Geometry: final body of the model. Coordinates: model frame, mm. A direction names the side the tool comes from. Coordinates: 2 decimals unless noted, no trailing zeros. Order: outer loops, then holes, each group sorted by start corner. A loop starts at its lowest first (then second) coordinate and runs counter-clockwise, first axis right, second up. Notation, with made-up numbers: (43, 74.25) - (68, 74.25) arc R25 ccw to (68, 113.25) - close; hole circle Ø4 at (64.5, -22.75). An arc over 180 degrees is marked (long way). Use a Markdown table: item, result. Add a question column.
```python
from build123d import *

# Parameters (mm, degrees)
ESBO_O1_W                = 77
ESBO_O1_H                = 57.5
RESSALTO_EXTRUS_O1_DEPTH = 2
ESBO_O2_W                = 7.7755798
ESBO_O2_H                = 8.143597904
ESBO_O2_W_2              = 8.031877
ESBO_O2_H_2              = 8.356901944
RESSALTO_EXTRUS_O2_DEPTH = 4
CASCA1_START             = -28.041915429
CASCA1_OUTLINE_W         = 6.031877
CASCA1_OUTLINE_H         = 4
CASCA1_OUTLINE_W_2       = 5.7755798
CASCA1_DEPTH             = 7.143597904
CASCA1_START_2           = -28.045301573
CASCA1_2_OUTLINE_W       = 6.031877
CASCA1_2_OUTLINE_H       = 4
CASCA1_2_DEPTH           = 7.356901944
ESBO_O3_R                = 1.331315802
ESBO_O3_R_2              = 1.316034484
ESBO_O3_R_3              = 1.436459579
ESBO_O3_R_4              = 1.302946869
CORTE_EXTRUS_O1_DEPTH    = 49.216309481


# Read off the part's stored shape, not the designer's step: Casca1
with BuildPart() as part:
    # Esboço1 → Ressalto-extrusão1 (new body)
    with BuildSketch(Plane(origin=(0, 0, 0), x_dir=(1, 0, 0), z_dir=(0, 1, 0))):
        Rectangle(ESBO_O1_W, ESBO_O1_H)
    extrude(amount=RESSALTO_EXTRUS_O1_DEPTH)

    # Esboço2 → Ressalto-extrusão2 (add)
    with BuildSketch(Plane(origin=(0, 2, 0), x_dir=(1, 0, 0), z_dir=(0, 1, 0))):
        with Locations((-23.313874366, 23.970116477)):
            Rectangle(ESBO_O2_W, ESBO_O2_H)
        with Locations((-5.149923387, 23.866850601)):
            Rectangle(ESBO_O2_W_2, ESBO_O2_H_2)
    extrude(amount=RESSALTO_EXTRUS_O2_DEPTH)

    # Casca1 outline → Casca1 (cut)
    with BuildSketch(Plane.XY.offset(CASCA1_START)):
        with Locations((-5.149923387, 3)):
            Rectangle(CASCA1_OUTLINE_W, CASCA1_OUTLINE_H)
        with Locations((-23.313874366, 3)):
            Rectangle(CASCA1_OUTLINE_W_2, CASCA1_OUTLINE_H)
    extrude(amount=CASCA1_DEPTH, mode=Mode.SUBTRACT)

    # Casca1 2 outline → Casca1 2 (cut)
    with BuildSketch(Plane.XY.offset(CASCA1_START_2)):
        with Locations((-5.149923387, 3)):
            Rectangle(CASCA1_2_OUTLINE_W, CASCA1_2_OUTLINE_H)
    extrude(amount=CASCA1_2_DEPTH, mode=Mode.SUBTRACT)

    # Esboço3 → Corte-extrusão1 (cut, through all)
    with BuildSketch(Plane(origin=(0, 2, 0), x_dir=(1, 0, 0), z_dir=(0, 1, 0))):
        with Locations(Location((33.733228093, -24.729326676, 0), (0, 0, 270))):
            Circle(ESBO_O3_R)
        with Locations(Location((34.598509611, 24.48523075, 0), (0, 0, 270))):
            Circle(ESBO_O3_R_2)
        with Locations(Location((-34.058204813, -24.729326676, 0), (0, 0, 270))):
            Circle(ESBO_O3_R_3)
        with Locations(Location((-34.058204813, 24.48523075, 0), (0, 0, 270))):
            Circle(ESBO_O3_R_4)
    extrude(amount=-CORTE_EXTRUS_O1_DEPTH, mode=Mode.SUBTRACT)


solid = part.part
```
1) Section C-C (x = -5). Return loops of the section in (y, z).
2) Section B-B (y = 4). Return loops of the section in (x, z).
3) Ray query, line 1 along X through (y, z) = (3.2, -25); line 2 along Z through (x, y) = (-23, 3.05); line 3 along Z through (x, y) = (-35, 1.35). Return the intervals inside material, ascending.
4) Section D-D (z = 18). Return loops of the section in (x, y).
5) Set-up query: faces 4 (the face through (-8.166, 3, -24)), 5 (the face through (-5, 5, -24)), 6 (the face through (-5, 4, -19.688)), 7 (the face through (-9.166, 4, -24)). Return all of +Z, -Z, +X, -X, +Y, -Y with unobstructed straight access to the full face (end or side cutting, diameter ignored); none if empty.
6) Pin query (flat end, axial travel): pin 1 (3.5 mm diameter, centred on x = -34.06, z = 24.73, fed in from -Y); pin 2 (8 mm diameter, centred on x = 20.5, z = 19, fed in from +Y); pin 3 (3 mm diameter, centred on y = 5, z = -18.5, fed in from -X). Return the tip coordinate at first contact, or that it passes through.
7) Draft query along X for faces 1 (the face through (-23, 3, -20.898)), 2 (the face through (-23, 4, -19.898)), 3 (the face through (-27.202, 4, -24)). Return one class per face: pulls with the +X half, pulls with the -X half, needs draft (parallel to the pull), parting line crosses it, or undercut.
8) Section A-A (z = -25). Return loops of the section in (x, y), then the cut area to 3 significant figures.
Values follow:
| question | item | result |
|---|---|---|
| 1 | outline | (0, -28.75) - (2, -28.75) - (2, -28.05) - (1, -28.05) - (1, -20.69) - (5, -20.69) - (5, -28.05) - (6, -28.05) - (6, -19.69) - (2, -19.69) - (2, 28.75) - (0, 28.75) - close |
| 2 | outline | (-27.2, -28.04) - (-26.2, -28.04) - (-26.2, -20.9) - (-20.43, -20.9) - (-20.43, -28.04) - (-19.43, -28.04) - (-19.43, -19.9) - (-27.2, -19.9) - close; (-9.17, -28.05) - (-8.17, -28.05) - (-8.17, -20.69) - (-2.13, -20.69) - (-2.13, -28.05) - (-1.13, -28.05) - (-1.13, -19.69) - (-9.17, -19.69) - close |
| 3 | line 1 | x = -27.2 to -26.2, -20.43 to -19.43, -9.17 to -8.17, -2.13 to -1.13 |
| 3 | line 2 | z = -20.9 to -19.9 |
| 3 | line 3 | z = -28.75 to -25.39, -23.58 to 23.64, 25.81 to 28.75 |
| 4 | outline | (-38.5, 0) - (38.5, 0) - (38.5, 2) - (-38.5, 2) - close |
| 5 | face 4 | none |
| 5 | face 5 | -Z |
| 5 | face 6 | +Z, +X, -X, +Y |
| 5 | face 7 | +Z, -Z, +Y |
| 6 | pin 1 | stops at y = 0 |
| 6 | pin 2 | stops at y = 2 |
| 6 | pin 3 | stops at x = -27.2 |
| 7 | face 1 | undercut |
| 7 | face 2 | needs draft |
| 7 | face 3 | pulls with the -X half |
| 8 | outline | (-38.5, 0) - (-35.26, 0) - (-35.26, 2) - (-38.5, 2) - close; (-32.86, 0) - (33.39, 0) - (33.39, 2) - (-1.13, 2) - (-1.13, 6) - (-9.17, 6) - (-9.17, 2) - (-19.43, 2) - (-19.43, 6) - (-27.2, 6) - (-27.2, 2) - (-32.86, 2) - close; (35.81, 0) - (38.5, 0) - (38.5, 2) - (35.81, 2) - close; hole (-26.2, 1) - (-20.43, 1) - (-20.43, 5) - (-26.2, 5) - close; hole (-8.17, 1) - (-2.13, 1) - (-2.13, 5) - (-8.17, 5) - close |
| 8 | area | 160 mm² |
